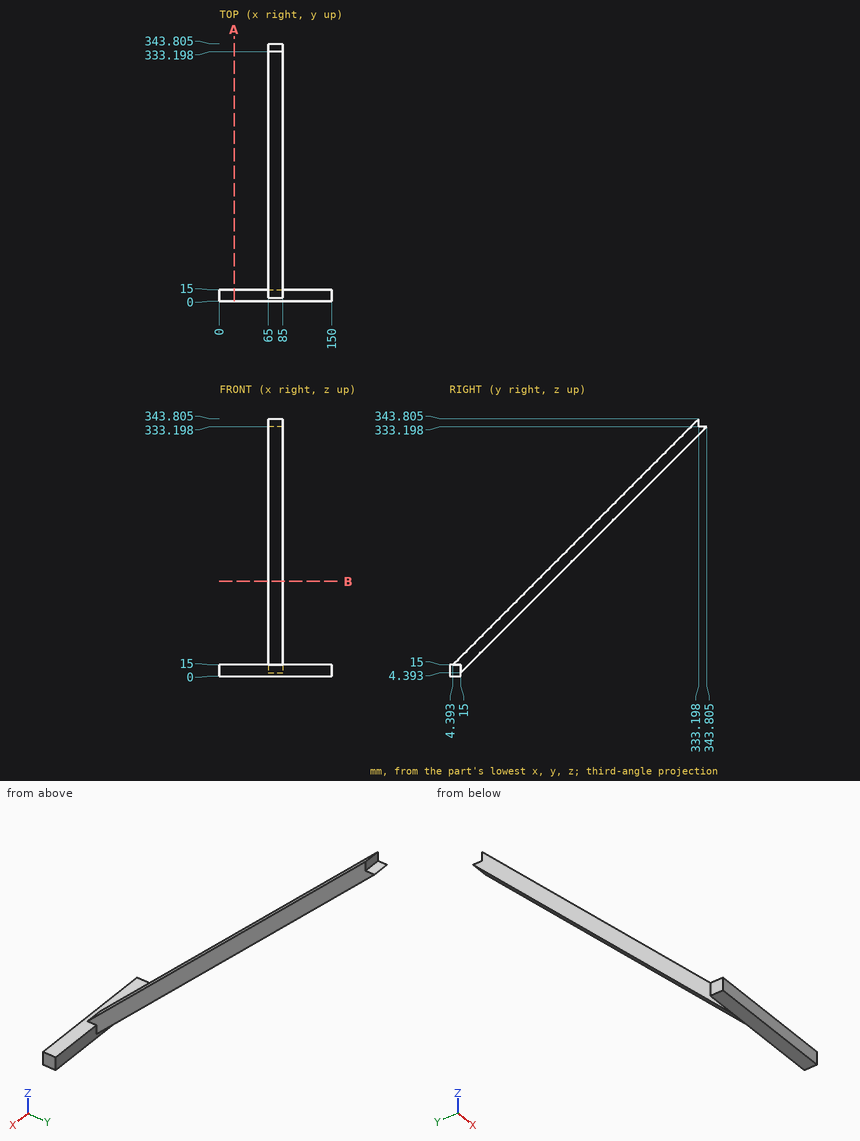
Study the drawing (mm; zero at the part's minimum x, y, z) and answer. Coordinates: 2 decimals unless noted, no trailing zeros. Loops run counter-clockwise (first coordinate to the right, second up) from the corner with the lowest first, then second, coordinate; pieces in that order, holes last. Notation, with made-up numbers: M 14,83 L 35,83 A14 cw 35,89 Z; hole C -9,30.5 d11. An arc over 180 degrees is marked long. Answer as a JSON object with one key per item and string values. Group by question number.
Item 1: Consider L1, parallel to X at y = 107, z = 102; L2, parallel to Z at x = 67.5, y = 274 (1 decimal); L3, parallel to Y at x = 71, z = 206 (1 decimal). Determine where each line is inside the solid, lowest interval first.
Item 2: Section B-B (z = 126.5) is taken. Write down the section's boundary in (x, y), and give its area (3 significant figures).
Item 3: Each of these flat-tipped pins is pushed along its axis until it touches: P1, Ø5.5, axis at x = 78, z = 337, coming from the +Y side; P2, Ø4.5, axis at x = 90.5, z = 4, coming from the +Y side; P3, Ø5.5, axis at x = 75.5, y = 338.5, coming from the +Z side. Where does it stop, or does it pass through?
Item 4: Section A-A (x = 19.5) is taken. Write down the section's boundary in (y, z), and give its area (3 significant figures).
Solved:
{
 "1": {"L1": "x = 65 to 85", "L2": "z = 263.4 to 284.6", "L3": "y = 195.4 to 216.6"},
 "2": {"outline": "M 65,115.89 L 85,115.89 L 85,137.11 L 65,137.11 Z", "area": "424 mm2"},
 "3": {"P1": "stops at y = 333.2", "P2": "stops at y = 15", "P3": "stops at z = 333.2"},
 "4": {"outline": "M 0,0 L 15,0 L 15,15 L 0,15 Z", "area": "225 mm2"}
}
